from build123d import *

# Parameters (mm, degrees)
SKETCH1_W           = 370
SKETCH1_H           = 280
SKETCH1_R           = 1.5
SKETCH1_R_2         = 1.569181713
SKETCH1_R_3         = 1.357318829
SKETCH1_R_4         = 1.322467774
SKETCH1_R_5         = 1
SKETCH1_W_2         = 230
SKETCH1_H_2         = 180
BOSS_EXTRUDE1_DEPTH = 4
SKETCH2_W           = 55
SKETCH2_H           = 12
CUT_EXTRUDE1_DEPTH  = 10
SKETCH3_R           = 1.5
CUT_EXTRUDE2_DEPTH  = 10
CUT_EXTRUDE3_DEPTH  = 10
FILLET3_R           = 5
FILLET4_R           = 5
FILLET5_R           = 5
FILLET6_R           = 5
FILLET7_R           = 5
FILLET8_R           = 5
FILLET9_R           = 5
SKETCH6_R           = 3.5
CUT_EXTRUDE4_DEPTH  = 10
SKETCH7_R           = 3.5
CUT_EXTRUDE5_DEPTH  = 10
SKETCH8_W           = 5
SKETCH8_H           = 3
SKETCH8_W_2         = 10
SKETCH8_H_2         = 15
SKETCH8_W_3         = 15
SKETCH8_H_3         = 5
SKETCH8_W_4         = 3
CUT_EXTRUDE6_DEPTH  = 10
SKETCH9_R           = 1.5
CUT_EXTRUDE7_DEPTH  = 10


with BuildPart() as part:
    # Sketch1 → Boss-Extrude1 (new body)
    with BuildSketch(Plane(origin=(0, 0, 0), x_dir=(1, 0, 0), z_dir=(0, 1, 0))):
        with Locations((185, 140)):
            Rectangle(SKETCH1_W, SKETCH1_H)
        with Locations((30, 274)):
            Circle(SKETCH1_R, mode=Mode.SUBTRACT)
        with Locations((50, 274)):
            Circle(SKETCH1_R_2, mode=Mode.SUBTRACT)
        with Locations((30, 6)):
            Circle(SKETCH1_R, mode=Mode.SUBTRACT)
        with Locations((50, 6)):
            Circle(SKETCH1_R, mode=Mode.SUBTRACT)
        with Locations((285.756924446, 273.985388104)):
            Circle(SKETCH1_R_3, mode=Mode.SUBTRACT)
        with Locations((305.756860025, 273.934625414)):
            Circle(SKETCH1_R, mode=Mode.SUBTRACT)
        with Locations((285.756860726, 6.001523901)):
            Circle(SKETCH1_R, mode=Mode.SUBTRACT)
        with Locations((305.756860025, 6.006818111)):
            Circle(SKETCH1_R_4, mode=Mode.SUBTRACT)
        with Locations((284, 145)):
            Circle(SKETCH1_R_5, mode=Mode.SUBTRACT)
        with Locations((284, 135)):
            Circle(SKETCH1_R_5, mode=Mode.SUBTRACT)
        with Locations((165, 140)):
            Rectangle(SKETCH1_W_2, SKETCH1_H_2, mode=Mode.SUBTRACT)
    extrude(amount=BOSS_EXTRUDE1_DEPTH)

    # Sketch2 → Cut-Extrude1 (cut)
    with BuildSketch(Plane(origin=(0, 4, 0), x_dir=(1, 0, 0), z_dir=(0, 1, 0))):
        with Locations((307.5, 224)):
            Rectangle(SKETCH2_W, SKETCH2_H)
    extrude(amount=-CUT_EXTRUDE1_DEPTH, mode=Mode.SUBTRACT)

    # Sketch3 → Cut-Extrude2 (cut)
    with BuildSketch(Plane(origin=(0, 4, 0), x_dir=(1, 0, 0), z_dir=(0, 1, 0))):
        with Locations((356, 147.5)):
            Circle(SKETCH3_R)
        with Locations((356, 132.5)):
            Circle(SKETCH3_R)
    extrude(amount=-CUT_EXTRUDE2_DEPTH, mode=Mode.SUBTRACT)

    # Sketch4 → Cut-Extrude3 (cut)
    with BuildSketch(Plane(origin=(0, 4, 0), x_dir=(1, 0, 0), z_dir=(0, 1, 0))):
        with BuildLine():
            Line((277.5, 266.5), (202.5, 266.5))
            ThreePointArc((202.5, 266.5), (201, 268), (202.5, 269.5))
            Line((202.5, 269.5), (277.5, 269.5))
            ThreePointArc((277.5, 269.5), (279, 268), (277.5, 266.5))
        make_face()
        with BuildLine():
            Line((277.5, 237), (202.5, 237))
            ThreePointArc((202.5, 237), (201, 238.5), (202.5, 240))
            Line((202.5, 240), (277.5, 240))
            ThreePointArc((277.5, 240), (279, 238.5), (277.5, 237))
        make_face()
    extrude(amount=-CUT_EXTRUDE3_DEPTH, mode=Mode.SUBTRACT)

    # Fillet3
    fillet3_edges = [part.edges().sort_by_distance(p)[0] for p in [
        (370, 2, 0),
    ]]
    fillet(fillet3_edges, radius=FILLET3_R)

    # Fillet4
    fillet4_edges = [part.edges().sort_by_distance(p)[0] for p in [
        (370, 2, -280),
    ]]
    fillet(fillet4_edges, radius=FILLET4_R)

    # Fillet5
    fillet5_edges = [part.edges().sort_by_distance(p)[0] for p in [
        (0, 2, 0),
    ]]
    fillet(fillet5_edges, radius=FILLET5_R)

    # Fillet6
    fillet6_edges = [part.edges().sort_by_distance(p)[0] for p in [
        (0, 2, -280),
    ]]
    fillet(fillet6_edges, radius=FILLET6_R)

    # Fillet7
    fillet7_edges = [part.edges().sort_by_distance(p)[0] for p in [
        (280, 2, -218),
    ]]
    fillet(fillet7_edges, radius=FILLET7_R)

    # Fillet8
    fillet8_edges = [part.edges().sort_by_distance(p)[0] for p in [
        (280, 2, -50),
    ]]
    fillet(fillet8_edges, radius=FILLET8_R)

    # Fillet9
    fillet9_edges = [part.edges().sort_by_distance(p)[0] for p in [
        (50, 2, -230),
        (50, 2, -50),
        (335, 2, -230),
        (335, 2, -218),
    ]]
    fillet(fillet9_edges, radius=FILLET9_R)

    # Sketch6 → Cut-Extrude4 (cut)
    with BuildSketch(Plane.XZ):
        with Locations((283.852252581, -253.25)):
            Circle(SKETCH6_R)
    extrude(amount=-CUT_EXTRUDE4_DEPTH, mode=Mode.SUBTRACT)

    # Sketch7 → Cut-Extrude5 (cut)
    with BuildSketch(Plane.XZ):
        with Locations((43.528330195, -36.357190156)):
            Circle(SKETCH7_R)
    extrude(amount=-CUT_EXTRUDE5_DEPTH, mode=Mode.SUBTRACT)

    # Sketch8 → Cut-Extrude6 (cut)
    with BuildSketch(Plane.XZ):
        with Locations((134.85877855, -14.984967273)):
            Rectangle(SKETCH8_W, SKETCH8_H)
        with Locations((134.85877855, -21.984967273)):
            Rectangle(SKETCH8_W, SKETCH8_H)
        with Locations((263.601107072, -30.863134191)):
            Rectangle(SKETCH8_W_2, SKETCH8_H_2)
        with Locations((311.102535039, -32.659137944)):
            Rectangle(SKETCH8_W, SKETCH8_H)
        with Locations((311.102535039, -39.659137944)):
            Rectangle(SKETCH8_W, SKETCH8_H)
        with Locations((307.626119627, -77.359497152)):
            Rectangle(SKETCH8_W_3, SKETCH8_H_3)
        with Locations((342.859262651, -236.259221691)):
            Rectangle(SKETCH8_W_4, SKETCH8_H_3)
        with Locations((349.859262651, -236.259221691)):
            Rectangle(SKETCH8_W_4, SKETCH8_H_3)
        with Locations((311.053880499, -174.438404524)):
            Rectangle(SKETCH8_W_3, SKETCH8_H_3)
    extrude(amount=-CUT_EXTRUDE6_DEPTH, mode=Mode.SUBTRACT)

    # Sketch9 → Cut-Extrude7 (cut)
    with BuildSketch(Plane.XZ):
        with Locations((25, -33)):
            Circle(SKETCH9_R)
        with Locations((25, -75)):
            Circle(SKETCH9_R)
    extrude(amount=-CUT_EXTRUDE7_DEPTH, mode=Mode.SUBTRACT)


solid = part.part
Geometry check sheet. Reference: the model listing, model coordinates, mm. Give positions to 0.01 mm unless a question says otherwise; leave off trailing zeros. Write each loop counter-clockwise with the first axis right and the second up, starting at its lowest first coordinate (ties: lowest second). Pieces come first, ordered by that corner, then holes. Notation, with made-up numbers: M 43.5,27 L 86.5,27 A17 cw 86.5,38 Z; hole C 84,43.25 d10. An arc over 180 degrees is marked long. One line per question, with ' | ' between items.
1. Mould release check, pull along X, two halves, no side actions. Record for faces 1 (the face through (182, 4, -235)), 2 (the face through (43.073, 1.972, -32.887)), 3 (the face through (285.467, 1.972, -256.355)): released by +X, released by -X, zero draft, split by the parting line, or undercut.
Ans:
face 1: zero draft | face 2: undercut | face 3: undercut
2. Cross-section at B-B (x = 127.5). Enter the section's corners in (y, z), plus the area to 3 significant figures.
Ans:
outline: M 0,-280 L 4,-280 L 4,-230 L 0,-230 Z; M 0,-50 L 4,-50 L 4,0 L 0,0 Z | area: 400 mm2
3. Cross-section at C-C (x = 235). Enter the section's corners in (y, z).
Ans:
outline: M 0,-280 L 4,-280 L 4,-269.5 L 0,-269.5 Z; M 0,-266.5 L 4,-266.5 L 4,-240 L 0,-240 Z; M 0,-237 L 4,-237 L 4,-230 L 0,-230 Z; M 0,-50 L 4,-50 L 4,0 L 0,0 Z
4. Gauge pin test, flat end, axial feed: pin 1 (1.8 mm diameter, centred on x = 305.76, z = -273.93, fed in from -Y). Record the tip position at first contact, or that the pin passes through.
Ans:
pin 1: through
5. Scan lines: line 1 along Z through (x, y) = (215, 3.2); line 2 along X through (y, z) = (3.1, -147.5); line 3 along Z through (x, y) = (315, 2.9). Record each from-to range of solid material in increasing order. Write a range as from..to.
Ans:
line 1: -280..-269.5, -266.5..-240, -237..-230, -50..0 | line 2: 0..50, 280..354.5, 357.5..370 | line 3: -280..-230, -218..-176.94, -171.94..-79.86, -74.86..0
6. Cross-section at A-A (z = -86). Enter the section's corners in (x, y).
Ans:
outline: M 0,0 L 50,0 L 50,4 L 0,4 Z; M 280,0 L 370,0 L 370,4 L 280,4 Z
